from build123d import *

# Parameters (mm, degrees)
BOSS_EXTRUDE2_DEPTH = 12.7
FILLET2_R           = 0.79375


with BuildPart() as part:
    # Sketch1 → Boss-Extrude2 (new body)
    with BuildSketch(Plane.XY):
        with BuildLine():
            Line((20.080431402, -6.524317111), (20.080431402, -18.716317111))
            Line((20.080431402, -18.716317111), (45.480431402, -18.716317111))
            Line((45.480431402, -18.716317111), (45.480431402, -19.510067111))
            Line((45.480431402, -19.510067111), (19.244107832, -19.510067111))
            Line((19.244107832, -19.510067111), (19.244107832, -18.721996551))
            Line((19.244107832, -18.721996551), (19.244107832, -6.524317111))
            ThreePointArc((19.244107832, -6.524317111), (0, 20.32), (-19.244107832, -6.524317111))
            Line((-19.244107832, -6.524317111), (-20.080431402, -6.524317111))
            ThreePointArc((-20.080431402, -6.524317111), (0, 21.11375), (20.080431402, -6.524317111))
        make_face()
        Polygon((-19.244107832, -6.524317111), (-19.244107832, -18.721996551), (-19.244107832, -19.510067111), (-45.480431402, -19.510067111), (-45.480431402, -18.716317111), (-20.080431402, -18.716317111), (-20.080431402, -6.524317111), align=None)
    extrude(amount=BOSS_EXTRUDE2_DEPTH)

    # Fillet2
    fillet2_edges = [part.edges().sort_by_distance(p)[0] for p in [
        (20.080431402, -18.716317111, 6.35),
        (19.244107832, -19.510067111, 6.35),
        (19.244107832, -6.524317111, 6.35),
        (-19.244107832, -6.524317111, 6.35),
        (-19.244107832, -19.510067111, 6.35),
        (-20.080431402, -18.716317111, 6.35),
        (-20.080431402, -6.524317111, 6.35),
        (20.080431402, -6.524317111, 6.35),
    ]]
    fillet(fillet2_edges, radius=FILLET2_R)


solid = part.part
Geometry: final body of the model. Coordinates: model frame, mm. A direction names the side the tool comes from. Give positions to 0.01 mm unless a question says otherwise; leave off trailing zeros. Order: outer loops, then holes, each group sorted by start corner. A loop starts at its lowest first (then second) coordinate and runs counter-clockwise, first axis right, second up. Notation, with made-up numbers: (-16, 58.5) -> (21, 58.5) arc R25 cw to (21, 71.5) -> close; hole circle Ø3 at (23, -0.75). An arc over 180 degrees is marked (long way). Answer as a JSON object with one key per item and string values.
Q1. Section A-A (y = -15). Output: boundary loops of the cut face in (x, z).
Entries:
{"outline": "(-20.08, 0) -> (-19.24, 0) -> (-19.24, 12.7) -> (-20.08, 12.7) -> close; (19.24, 0) -> (20.08, 0) -> (20.08, 12.7) -> (19.24, 12.7) -> close"}
Q2. Draft query along X for faces 1 (the flat face through (19.244, -13, 6)), 2 (the flat face through (-20.08, -12, 6)), 3 (the flat face through (-20, -5, 0)). Return one class per face: released by +X, released by -X, zero draft, split by the parting line, or undercut.
Entries:
{"face 1": "undercut", "face 2": "released by -X", "face 3": "zero draft"}
Q3. Section B-B (z = 9). Output: boundary loops of the cut face in (x, y), plus the area to 3 significant figures.
Entries:
{"outline": "(-45.48, -19.51) -> (-20.04, -19.51) arc R0.79 ccw to (-19.24, -18.72) -> (-19.24, -6.65) arc R0.79 ccw to (-19.28, -6.4) arc R20.32 cw (long way) to (19.28, -6.4) arc R0.79 ccw to (19.24, -6.65) -> (19.24, -18.72) arc R0.79 ccw to (20.04, -19.51) -> (45.48, -19.51) -> (45.48, -18.72) -> (20.87, -18.72) arc R0.79 cw to (20.08, -17.92) -> (20.08, -6.65) arc R0.79 cw to (20.12, -6.41) arc R21.11 ccw (long way) to (-20.12, -6.41) arc R0.79 cw to (-20.08, -6.65) -> (-20.08, -17.92) arc R0.79 cw to (-20.87, -18.72) -> (-45.48, -18.72) -> close", "area": "124 mm^2"}
Q4. First-contact query: pin 1 (3 mm diameter, centred on x = 14.5, y = 14, fed in from +Z); pin 2 (2 mm diameter, centred on y = -7, z = 2, fed in from +X); pin 3 (6.5 mm diameter, centred on x = -27, z = 5, fed in from +Y); pin 4 (4 mm diameter, centred on x = 5, z = 8, fed in from +Y). Flat tips, straight axial feed; report the tip coordinate or a pass-through.
Entries:
{"pin 1": "stops at z = 12.7", "pin 2": "stops at x = 20.24", "pin 3": "stops at y = -18.72", "pin 4": "stops at y = 20.9"}
Q5. Material intervals for probe 1 along X at (y, z) = (0, 3.75); probe 2 along X at (y, z) = (-7.5, 8); probe 3 along Y at (x, z) = (31, 3.5), sorted ascending.
Entries:
{"probe 1": "x = -21.11 to -20.32, 20.32 to 21.11", "probe 2": "x = -20.08 to -19.24, 19.24 to 20.08", "probe 3": "y = -19.51 to -18.72"}
Q6. Access query for faces 4 (the flat face through (-19.244, -13, 6)), 5 (the flat face through (20.08, -12, 6)), 6 (the flat face through (-33, -19.51, 6)). Directions: +Z, -Z, +X, -X, +Y, -Y. A direction counts if a zero-diameter tool reaches every point of the face in a straight line with its end or side. Return the directions, or none.
Entries:
{"face 4": "+Z, -Z, -Y", "face 5": "+Z, -Z, +X", "face 6": "+Z, -Z, +X, -X, -Y"}
Q7. Section C-C (y = 0). Output: boundary loops of the cut face in (x, z).
Entries:
{"outline": "(-21.11, 0) -> (-20.32, 0) -> (-20.32, 12.7) -> (-21.11, 12.7) -> close; (20.32, 0) -> (21.11, 0) -> (21.11, 12.7) -> (20.32, 12.7) -> close"}
Q8. Section D-D (x = 2.5). Output: boundary loops of the cut face in (y, z).
Entries:
{"outline": "(20.17, 0) -> (20.97, 0) -> (20.97, 12.7) -> (20.17, 12.7) -> close"}
